Design review of the part built by this model. Coordinates are the model's own, in mm. Face numbers are marked on the shaded views. A direction names the side the tool comes from. Give positions to 0.01 mm unless a question says otherwise; leave off trailing zeros. Loops run counter-clockwise (first coordinate to the right, second up) from the corner with the lowest first, then second, coordinate; pieces in that order, holes last. Notation, with made-up numbers: M 14,-7 L 61,-7 A26 cw 61,28 Z; hole C 23,83.25 d4. An arc over 180 degrees is marked long. Use a Markdown table: item, result. Add a question column.
(1) Add section C-C, the plane y = 106.5. Give the boundary of the cut face in (x, z), then the cut area to 3 significant figures.
(2) Add section A-A, the plane x = 244. Give the boundary of the cut face in (y, z), then the cut area to 3 significant figures.
(3) Add section D-D, the plane z = 22. Give the boundary of the cut face in (x, y), then the cut area to 3 significant figures.
(4) For probe 1 along Y at (x, z) = (270.75, 30); probe 2 along Y at (x, z) = (272.8, 30); probe 3 along Z at (x, y) = (270, 181), list the stretches that pass through material, from the lowest coordinate up.
(5) Draft analysis for pull direction Z (two halves, no side actions). For the marked faces 1, 2 and 3, state which applies: pulls with the +Z half, pulls with the -Z half, needs draft (parallel to the pull), parting line crosses it, or undercut.
(6) For the marked faces 4 and 5, list the 3-axis set-ups (+Z, -Z, +X, -X, +Y, -Y) from which the entire face can be reached by the end or side of a thin tool; tool diameter is ignored.
(7) Insertion check: pin 1 Ø4 at (x, y) = (170.5, 163.5) entering from -Z; pin 2 Ø22.5 at (y, z) = (125, 30) entering from -X; pin 3 Ø4 at (y, z) = (116.25, 30) entering from +X; pin 4 Ø22.5 at (y, z) = (130.5, 34) entering from -X. Each pin has a flat end and moves straight along its axis. Give the tip position at first contact, or say it passes through.
(8) Add section B-B, the plane y = 168. Give the boundary of the cut face in (x, z), then the cut area to 3 significant figures.
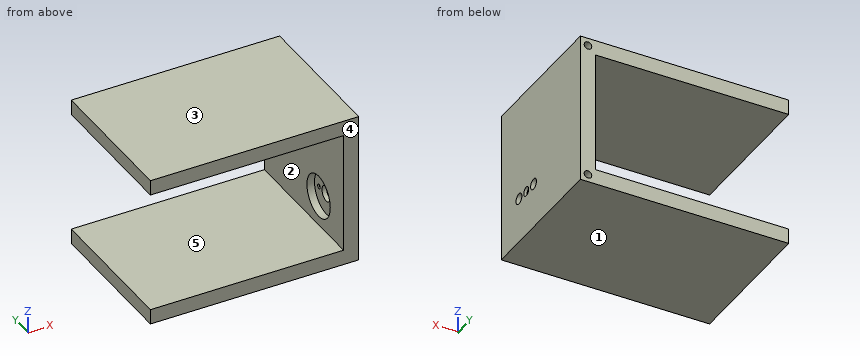
Autodesk Inventor part; units mm, degrees
ref_plane "YZ Plane" through (0, 0, 0) normal (1, 0, 0) x (0, 1, 0)
ref_plane "XZ Plane" through (0, 0, 0) normal (0, 1, 0) x (-1, 0, 0)
ref_plane "XY Plane" through (0, 0, 0) normal (0, 0, 1) x (1, 0, 0)
sketch "Sketch1" plane through (0, 0, 0) normal (0, 0, 1) x (1, 0, 0)
  line L0 (0, 0) -> (275, 0)
  line L1 (275, 0) -> (275, 200)
  line L2 (275, 200) -> (0, 200)
  line L3 (0, 200) -> (0, 0)
  dimension "d0" = 275
  dimension "d1" = 200
extrude "Extrusion1" add sketch "Sketch1" along normal blind 20
sketch "Sketch3" plane through (0, 0, 20) normal (0, 0, 1) x (1, 0, 0)
  line L0 (275, 0) -> (275, 200)
  line L1 (0, 200) -> (275, 200)
  line L2 (275, 200) -> (275, 0)
  line L3 (275, 0) -> (0, 0)
  line L4 (0, 0) -> (0, 200)
  point P0 (0, 0)
extrude "Extrusion3" add sketch "Sketch3" along normal blind 80
sketch "Sketch4" plane through (0, 0, 0) normal (0, -1, 0) x (1, 0, 0)
  circle A0 centre (47.5, 50) radius 17.5
  circle A1 centre (227.5, 50) radius 17.5
  line L0 (47.5, 50) -> (227.5, 50) construction
  line L1 (0, 0) -> (0, 100)
  line L2 (0, 100) -> (275, 100)
  point P0 (0, 50)
  point P1 (137.5, 50)
  point P2 (137.5, 100)
  dimension "d10" = 35
  dimension "d11" = 35
  dimension "d12" = 180
extrude "Extrusion4" cut sketch "Sketch4" against normal blind 100 contours A0
sketch "Sketch5" plane through (0, 200, 0) normal (0, 1, 0) x (1, 0, 0)
  line L0 (275, 0) -> (0, 0)
  line L1 (0, 0) -> (0, -100)
  line L2 (275, -100) -> (0, -100)
  line L3 (275, 0) -> (275, -100)
  line L4 (265, -90) -> (10, -90)
  line L5 (10, -90) -> (10, -10)
  line L6 (10, -10) -> (265, -10)
  line L7 (265, -10) -> (265, -90)
  point P0 (0, 0)
  dimension "d15" = 10
extrude "Extrusion5" cut sketch "Sketch5" against normal blind 190 contours L4 L5 L6 L7
sketch "Sketch6" plane through (0, 0, 0) normal (-1, 0, 0) x (0, 0, 1)
  line L0 (0, 200) -> (100, 200)
  line L1 (0, 200) -> (0, 0)
  line L2 (100, 200) -> (0, 200)
  line L3 (0, 200) -> (0, 190)
  line L4 (0, 190) -> (100, 190)
  line L5 (100, 190) -> (100, 200)
  dimension "d18" = 10
extrude "Extrusion6" cut sketch "Sketch6" against normal through all
sketch "Sketch7" plane through (0, 190, 100) normal (0, 1, 0) x (1, 0, 0)
  line L0 (275, 100) -> (275, 0) construction
  line L1 (0, 100) -> (275, 100) construction
  line L2 (0, 0) -> (0, 100) construction
  line L3 (275, 0) -> (0, 0) construction
  line L4 (265, 10) -> (265, 90) construction
  line L5 (10, 10) -> (265, 10) construction
  line L6 (10, 90) -> (10, 10) construction
  line L7 (265, 90) -> (10, 90) construction
  line L8 (270, 5) -> (270, 95) construction
  line L9 (270, 95) -> (5, 95) construction
  line L10 (5, 95) -> (5, 5) construction
  line L11 (5, 5) -> (270, 5) construction
  circle A0 centre (270, 5) radius 2.5
  circle A1 centre (270, 95) radius 2.5
  circle A2 centre (5, 95) radius 2.5
  circle A3 centre (5, 5) radius 2.5
  point P0 (0, 100)
  dimension "d21" = 5
  dimension "d22" = 5
  dimension "d23" = 5
  dimension "d24" = 5
  dimension "d25" = 5
extrude "Extrusion7" cut sketch "Sketch7" against normal blind 25
sketch "Sketch8" plane through (0, 0, 0) normal (0, -1, 0) x (1, 0, 0)
  line L0 (82, 15) -> (85, 15)
  line L1 (85, 15) -> (85, 35)
  line L2 (85, 35) -> (82, 35)
  line L3 (82, 35) -> (82, 15)
  line L4 (0, 0) -> (0, 100)
  line L5 (0, 0) -> (275, 0)
  line L6 (97, 15) -> (97, 35)
  line L7 (97, 35) -> (94, 35)
  line L8 (94, 35) -> (94, 15)
  line L9 (94, 15) -> (97, 15)
  line L10 (109, 15) -> (109, 35)
  line L11 (109, 35) -> (106, 35)
  line L12 (106, 35) -> (106, 15)
  line L13 (106, 15) -> (109, 15)
  line L14 (121, 15) -> (121, 35)
  line L15 (121, 35) -> (118, 35)
  line L16 (118, 35) -> (118, 15)
  line L17 (118, 15) -> (121, 15)
  line L18 (133, 15) -> (133, 35)
  line L19 (133, 35) -> (130, 35)
  line L20 (130, 35) -> (130, 15)
  line L21 (130, 15) -> (133, 15)
  line L22 (145, 15) -> (145, 35)
  line L23 (145, 35) -> (142, 35)
  line L24 (142, 35) -> (142, 15)
  line L25 (142, 15) -> (145, 15)
  line L26 (157, 15) -> (157, 35)
  line L27 (157, 35) -> (154, 35)
  line L28 (154, 35) -> (154, 15)
  line L29 (154, 15) -> (157, 15)
  line L30 (169, 15) -> (169, 35)
  line L31 (169, 35) -> (166, 35)
  line L32 (166, 35) -> (166, 15)
  line L33 (166, 15) -> (169, 15)
  line L34 (181, 15) -> (181, 35)
  line L35 (181, 35) -> (178, 35)
  line L36 (178, 35) -> (178, 15)
  line L37 (178, 15) -> (181, 15)
  line L38 (193, 15) -> (193, 35)
  line L39 (193, 35) -> (190, 35)
  line L40 (190, 35) -> (190, 15)
  line L41 (190, 15) -> (193, 15)
  line L42 (205, 15) -> (205, 35)
  line L43 (205, 35) -> (202, 35)
  line L44 (202, 35) -> (202, 15)
  line L45 (202, 15) -> (205, 15)
  line L46 (217, 15) -> (217, 35)
  line L47 (217, 35) -> (214, 35)
  line L48 (214, 35) -> (214, 15)
  line L49 (214, 15) -> (217, 15)
  line L50 (229, 15) -> (229, 35)
  line L51 (229, 35) -> (226, 35)
  line L52 (226, 35) -> (226, 15)
  line L53 (226, 15) -> (229, 15)
  line L54 (241, 15) -> (241, 35)
  line L55 (241, 35) -> (238, 35)
  line L56 (238, 35) -> (238, 15)
  line L57 (238, 15) -> (241, 15)
  dimension "d28" = 3
  dimension "d29" = 20
  dimension "d30" = 82
  dimension "d31" = 15
  dimension "d34" = 12
extrude "Extrusion8" cut sketch "Sketch8" against normal through all
sketch "Sketch2" plane through (275, 0, 100) normal (1, 0, 0) x (0, 0, -1)
  circle A0 centre (70, 125) radius 3
  line L0 (100, 0) -> (0, 0)
  line L1 (100, 0) -> (100, 190)
  dimension "d4" = 6
  dimension "d45" = 125
  dimension "d46" = 30
extrude "Extrusion2" cut sketch "Sketch2" against normal through all
sketch "Sketch10" plane through (0, 190, 100) normal (0, 1, 0) x (1, 0, 0)
  line L0 (0, 100) -> (275, 100)
  line L1 (275, 0) -> (0, 0)
  line L2 (0, 100) -> (137.5, 100)
  line L3 (137.5, 100) -> (137.5, 0)
  line L4 (137.5, 0) -> (0, 0)
  line L5 (0, 0) -> (0, 100)
extrude "Extrusion10" cut sketch "Sketch10" against normal through all
sketch "Sketch12" plane through (0, 0, 100) normal (0, 0, 1) x (1, 0, 0)
  line L0 (137.5, 0) -> (275, 0)
  line L1 (275, 0) -> (275, 190)
  line L2 (137.5, 0) -> (275, 0)
  line L3 (275, 0) -> (275, 95)
  line L4 (275, 95) -> (137.5, 95)
  line L5 (137.5, 95) -> (137.5, 0)
  point P0 (0, 0)
  dimension "d52" = 95
extrude "Extrusion11" cut sketch "Sketch12" against normal through all
sketch "Sketch13" plane through (265, 190, 10) normal (-1, 0, 0) x (0, 0, 1)
  circle A0 centre (20, -56.25) radius 1.5
  circle A1 centre (20, -73.75) radius 1.5
  line L0 (20, -56.25) -> (20, -73.75) construction
  circle A2 centre (20, -65) radius 3
  point P0 (-10, -190)
  dimension "d53" = 3
  dimension "d54" = 3
  dimension "d55" = 17.5
extrude "Extrusion12" cut sketch "Sketch13" against normal through all contours A0 | A1
sketch "Sketch14" plane through (265, 190, 10) normal (-1, 0, 0) x (0, 0, 1)
  circle A0 centre (20, -65) radius 14
  circle A1 centre (20, -65) radius 3
  point P0 (-10, -190)
  dimension "d58" = 28
extrude "Extrusion13" cut sketch "Sketch14" against normal blind 5
sketch "Sketch15" plane through (270, 125, 30) normal (-1, 0, 0) x (0, 0, 1)
  circle A0 centre (0, 0) radius 3
  circle A1 centre (0, 0) radius 5
  point P0 (-30, -125)
  dimension "d61" = 10
extrude "Extrusion14" cut sketch "Sketch15" against normal blind 3
sketch "Sketch16" plane through (275, 190, 100) normal (1, 0, 0) x (0, 0, -1)
  circle A0 centre (70, -56.25) radius 1.5
  circle A1 centre (70, -73.75) radius 1.5
  circle A2 centre (70, -56.25) radius 1.5
  circle A3 centre (70, -56.25) radius 3.5
  circle A4 centre (70, -73.75) radius 1.5
  circle A5 centre (70, -73.75) radius 3.5
  point P0 (100, -190)
  dimension "d64" = 7
  dimension "d65" = 7
extrude "Extrusion15" cut sketch "Sketch16" against normal blind 4 contours A0 | A1 | A3 | A5
properties part number "HA005" material "ABS Plastic"
Established:
| question | item | result |
|---|---|---|
| 1 | outline | M 137.5,0 L 275,0 L 275,100 L 137.5,100 L 137.5,90 L 265,90 L 265,10 L 137.5,10 Z |
| 1 | area | 3,550 mm^2 |
| 2 | outline | M 95,0 L 190,0 L 190,10 L 95,10 Z; M 95,90 L 190,90 L 190,100 L 95,100 Z |
| 2 | area | 1,900 mm^2 |
| 3 | outline | M 265,95 L 275,95 L 275,190 L 265,190 L 265,136.49 L 270,136.49 L 270,113.51 L 265,113.51 Z |
| 3 | area | 835 mm^2 |
| 4 | probe 1 | 95 to 114.75, 117.75 to 120, 130 to 132.25, 135.25 to 190 |
| 4 | probe 2 | 95 to 112.75, 119.75 to 120, 130 to 130.25, 137.25 to 190 |
| 4 | probe 3 | 0 to 2.5, 7.5 to 92.5, 97.5 to 100 |
| 5 | face 1 | pulls with the -Z half |
| 5 | face 2 | undercut |
| 5 | face 3 | pulls with the +Z half |
| 6 | face 4 | +Z, -Z, +X, -X, -Y |
| 6 | face 5 | -X, +Y, -Y |
| 7 | pin 1 | z = 0 |
| 7 | pin 2 | x = 270 |
| 7 | pin 3 | x = 271 |
| 7 | pin 4 | x = 265 |
| 8 | outline | M 137.5,0 L 275,0 L 275,100 L 137.5,100 L 137.5,90 L 265,90 L 265,10 L 137.5,10 Z; hole C 270,5 d5; hole C 270,95 d5 |
| 8 | area | 3,510 mm^2 |
